```python
from build123d import *

# Parameters (mm, degrees)
SKETCH1_R           = 2
SKETCH1_R_2         = 6.35
SKETCH1_R_3         = 3.175
BOSS_EXTRUDE1_DEPTH = 3.175


with BuildPart() as part:
    # Sketch1 → Boss-Extrude1 (new body)
    with BuildSketch(Plane(origin=(0, 0, 0), x_dir=(0, 0, -1), z_dir=(1, 0, 0))):
        Polygon((-12.7, 101.6), (57.15, 101.6), (57.15, 31.75), (12.7, -12.7), (-12.7, -12.7), align=None)
        with Locations((36.0553, 53.601042741)):
            Circle(SKETCH1_R, mode=Mode.SUBTRACT)
        Circle(SKETCH1_R_2, mode=Mode.SUBTRACT)
        with Locations((0, 88.9)):
            Circle(SKETCH1_R_3, mode=Mode.SUBTRACT)
        with Locations((44.45, 88.9)):
            Circle(SKETCH1_R_3, mode=Mode.SUBTRACT)
        with Locations((0, 53.601042741)):
            Circle(SKETCH1_R_3, mode=Mode.SUBTRACT)
    extrude(amount=BOSS_EXTRUDE1_DEPTH)


solid = part.part
```
Model file for the job. Use its own axes, mm. Give positions to 0.01 mm unless a question says otherwise; leave off trailing zeros. Loops run counter-clockwise (first coordinate to the right, second up) from the corner with the lowest first, then second, coordinate; pieces in that order, holes last. Notation, with made-up numbers: (-27, -7.5) - (10, -7.5) arc R21 cw to (10, 4.5) - close; hole circle Ø1 at (31, 65.5). An arc over 180 degrees is marked (long way). One line per item, written item: value. Start each with the question number.
1. Slice it at A-A (z = 0). List the corners of the cut face in (x, y) (3 decimals), plus the area to 3 significant figures.
2. Probe L1, parallel to Y at x = 2.2, z = 0 (3 decimals); L2, parallel to Z at x = 0.6, y = 87; L3, parallel to Y at x = 1.55, z = -2.5. List the from-to ranges inside material, lowest first. Write a range as from..to.
3. Slice it at D-D (z = -44.45). List the corners of the cut face in (x, y) (3 decimals).
4. Pull direction Z, two halves, no side cores. Call faces 1 (the cylindrical face through (1.565, 56.278, -1.707)), 2 (the flat face through (2, -12.7, 0)), 3 (the flat face through (1.6, 9.8, -35.2)): pulls with the +Z half, pulls with the -Z half, needs draft (parallel to the pull), parting line crosses it, or undercut.
5. Slice it at B-B (y = 0). List the corners of the cut face in (x, z) (3 decimals), plus the area to 3 significant figures.
6. Slice it at C-C (y = 88.9). List the corners of the cut face in (x, z) (3 decimals), plus the area to 3 significant figures.
Solution:
1. outline: (0, -12.7) - (3.175, -12.7) - (3.175, -6.35) - (0, -6.35) - close; (0, 6.35) - (3.175, 6.35) - (3.175, 50.426) - (0, 50.426) - close; (0, 56.776) - (3.175, 56.776) - (3.175, 85.725) - (0, 85.725) - close; (0, 92.075) - (3.175, 92.075) - (3.175, 101.6) - (0, 101.6) - close
1. area: 282 mm^2
2. L1: y = -12.7..-6.35, 6.35..50.426, 56.776..85.725, 92.075..101.6
2. L2: z = -57.15..-46.99, -41.91..-2.54, 2.54..12.7
2. L3: y = -12.7..-5.84, 5.84..51.64, 55.56..86.94, 90.86..101.6
3. outline: (0, 19.05) - (3.175, 19.05) - (3.175, 85.725) - (0, 85.725) - close; (0, 92.075) - (3.175, 92.075) - (3.175, 101.6) - (0, 101.6) - close
4. face 1: undercut
4. face 2: needs draft
4. face 3: pulls with the -Z half
5. outline: (0, -25.4) - (3.175, -25.4) - (3.175, -6.35) - (0, -6.35) - close; (0, 6.35) - (3.175, 6.35) - (3.175, 12.7) - (0, 12.7) - close
5. area: 80.6 mm^2
6. outline: (0, -57.15) - (3.175, -57.15) - (3.175, -47.625) - (0, -47.625) - close; (0, -41.275) - (3.175, -41.275) - (3.175, -3.175) - (0, -3.175) - close; (0, 3.175) - (3.175, 3.175) - (3.175, 12.7) - (0, 12.7) - close
6. area: 181 mm^2
